The model under review builds one solid part; all positions refer to its coordinate system, in mm. A direction names the side the tool comes from. Coordinates: 2 decimals unless noted, no trailing zeros. Order: outer loops, then holes, each group sorted by start corner. A loop starts at its lowest first (then second) coordinate and runs counter-clockwise, first axis right, second up.
from build123d import *

# Parameters (mm, degrees)
PAD_DEPTH = 2.5


with BuildPart() as part:
    # Sketch → Pad (new body)
    with BuildSketch(Plane.XY):
        with BuildLine():
            Line((-3.5, 1e-05), (-5, 0))
            Line((-5, 0), (-5, 10))
            Line((-5, 10), (-5, 14))
            Line((-5, 14), (5, 14))
            Line((5, 14), (5, 10.017754))
            ThreePointArc((3.940727, 6.163882), (4.737162, 8.017486), (5, 10.017754))
            ThreePointArc((3.940727, 6.163882), (2.660853, 3.199304), (2.223533, 0))
            Line((0.995967, 0), (2.223533, 0))
            ThreePointArc((2.889985, 6.798595), (1.478319, 3.528746), (0.995967, 0))
            ThreePointArc((2.889985, 6.798595), (3.553374, 8.342393), (3.772469, 10.008344))
            Line((3.772469, 10.008344), (2.542243, 10))
            ThreePointArc((2.219305, 8.420788), (2.460682, 9.194053), (2.542243, 10))
            ThreePointArc((2.219305, 8.420788), (0.932219, 4.297526), (0.497311, 0))
            Line((0.497311, 0), (-1.002689, 0))
            ThreePointArc((0.839722, 9.009643), (-0.537369, 4.598047), (-1.002689, 0))
            ThreePointArc((0.839722, 9.009643), (0.991094, 9.494574), (1.042243, 10))
            Line((1.042243, 10), (-0.431539, 10))
            ThreePointArc((-0.502671, 9.335096), (-0.449373, 9.665651), (-0.431539, 10))
            ThreePointArc((-0.502671, 9.335096), (-1.250966, 4.694181), (-1.501344, 0))
            Line((-3.001344, 0), (-1.501344, 0))
            ThreePointArc((-1.968725, 9.652406), (-2.742455, 4.853742), (-3.001344, 0))
            ThreePointArc((-1.968725, 9.652406), (-1.940862, 9.825211), (-1.931539, 10))
            Line((-3.5, 10), (-1.931539, 10))
            Line((-3.5, 10), (-3.5, 1e-05))
        make_face()
    pad = extrude(amount=PAD_DEPTH)

    # Mirrored: Pad across Sketch H_Axis
    add(pad.mirror(Plane.ZX))


solid = part.part
(1) Consider section D-D (y = 8). Give the boundary of the cut face in (x, z).
(2) The part is to be moulded in two halves that separate along Y. For faces 3 (the face through (0, 0, 2.5)), 4 (the face through (0, 14, 1)), 5 (the face through (4.73, -7.99, 1.23)), 6 (the face through (0, -10, 1)), say which applies: +Y half, -Y half, draft (parallel to the pull), parting line (faces both ways), or undercut.
(3) Wall thickness on line 1 (X direction, y = -0.25, z = 1.65); line 2 (Y direction, x = -3.25, z = 1.8); line 3 (Y direction, x = 3.25, z = 1.5): over which ranges is each line inside the solid? List them lowest first.
(4) Consider section A-A (y = -1). Give the boundary of the cut face in (x, z), then the cut area to 3 significant figures.
(5) Tool access review of faces 1 (the face through (3.547, 8.32, 1.232)), 2 (the face through (-5, -7, 1)): name each direction out of +Z, -Z, +X, -X, +Y, -Y from which nothing blocks a thin tool from reaching the whole face with its end or side.
(6) Insertion check: pin 1 Ø1 at (y, z) = (-4, 2) entering from +X; pin 2 Ø2 at (x, y) = (1.5, 0.5) entering from -Z; pin 3 Ø0.8 at (y, z) = (6.5, 1.5) entering from +X; pin 4 Ø1.2 at (y, z) = (-6.5, 1.5) entering from +X. Each pin has a flat end and moves straight along its axis. Give the tip position at first contact, or say it passes through.
(7) Consider section B-B (x = -0.75). Give the boundary of the cut face in (y, z), then the cut area to 3 significant figures.
Findings:
1. outline: (-5, 0) - (-3.5, 0) - (-3.5, 2.5) - (-5, 2.5) - close; (-2.29, 0) - (-0.77, 0) - (-0.77, 2.5) - (-2.29, 2.5) - close; (0.44, 0) - (2.04, 0) - (2.04, 2.5) - (0.44, 2.5) - close; (3.45, 0) - (4.73, 0) - (4.73, 2.5) - (3.45, 2.5) - close
2. face 3: draft
2. face 4: +Y half
2. face 5: undercut
2. face 6: undercut
3. line 1: x = -5 to -3.5, -3 to -1.5, -1 to 0.5, 1 to 2.23
3. line 2: y = -14 to -10, 10 to 14
3. line 3: y = -14 to -10, -7.49 to -4.84, 4.84 to 7.49, 10 to 14
4. outline: (-5, 0) - (-3.5, 0) - (-3.5, 2.5) - (-5, 2.5) - close; (-2.99, 0) - (-1.49, 0) - (-1.49, 2.5) - (-2.99, 2.5) - close; (-0.98, 0) - (0.52, 0) - (0.52, 2.5) - (-0.98, 2.5) - close; (1.03, 0) - (2.27, 0) - (2.27, 2.5) - (1.03, 2.5) - close
4. area: 14.3 mm2
5. face 1: +Z, -Z
5. face 2: +Z, -Z, -X, +Y, -Y
6. pin 1: stops at x = 3.11
6. pin 2: stops at z = 0
6. pin 3: stops at x = 4.33
6. pin 4: stops at x = 4.42
7. outline: (-14, 0) - (-8.11, 0) - (-8.11, 2.5) - (-14, 2.5) - close; (-3.4, 0) - (3.4, 0) - (3.4, 2.5) - (-3.4, 2.5) - close; (8.11, 0) - (14, 0) - (14, 2.5) - (8.11, 2.5) - close
7. area: 46.4 mm2
